The model under review builds one solid part; all positions refer to its coordinate system, in mm. A direction names the side the tool comes from. Give positions to 0.01 mm unless a question says otherwise; leave off trailing zeros. Order: outer loops, then holes, each group sorted by start corner. A loop starts at its lowest first (then second) coordinate and runs counter-clockwise, first axis right, second up. Notation, with made-up numbers: (-33, -3) - (14, -3) arc R31 ccw to (14, 24) - close; hole circle Ø11 at (-38.75, -7). An arc over 180 degrees is marked (long way). Use CSV: the item, a comma, the result in double quotes.
```python
from build123d import *

# Parameters (mm, degrees)
SKETCH1_W           = 56.05
SKETCH1_H           = 61.05
SKETCH1_W_2         = 50.05
SKETCH1_H_2         = 55.05
SKETCH1_W_3         = 44.05
SKETCH1_H_3         = 49.05
BOSS_EXTRUDE1_DEPTH = 3
SKETCH1_3_W         = 56.05
SKETCH1_3_H         = 61.05
SKETCH1_3_W_2       = 50.05
SKETCH1_3_H_2       = 55.05
SKETCH1_3_W_3       = 44.05
SKETCH1_3_H_3       = 49.05
BOSS_EXTRUDE2_DEPTH = 15
SKETCH1_4_W         = 50.05
SKETCH1_4_H         = 55.05
SKETCH1_4_W_2       = 44.05
SKETCH1_4_H_2       = 49.05
BOSS_EXTRUDE3_DEPTH = 18
FILLET1_R           = 2
SKETCH2_R           = 13.25
CUT_EXTRUDE1_DEPTH  = 19
SKETCH2_9_R         = 2.825
SKETCH2_9_R_2       = 1.6
SKETCH2_9_R_3       = 13.25
CUT_EXTRUDE2_DEPTH  = 3
CUT_EXTRUDE3_START  = -3
SKETCH2_10_R        = 1.6
SKETCH2_10_W        = 13
SKETCH2_10_H        = 10.44
SKETCH2_10_H_2      = 1
SKETCH2_10_W_2      = 0.1
SKETCH2_10_H_3      = 11.1
CUT_EXTRUDE3_DEPTH  = 16
SKETCH5_W           = 44.05
SKETCH5_H           = 49.05
CUT_EXTRUDE4_DEPTH  = 1.6
SKETCH2_11_W        = 2.25
SKETCH2_11_H        = 0.408076211
SKETCH2_11_W_2      = 1.5
SKETCH2_11_H_2      = 2.5
CUT_EXTRUDE5_DEPTH  = 1.6


with BuildPart() as part:
    # Sketch1 → Boss-Extrude1 (new body)
    with BuildSketch(Plane(origin=(0, 0, 0), x_dir=(1, 0, 0), z_dir=(0, 1, 0))):
        Rectangle(SKETCH1_W, SKETCH1_H)
        Rectangle(SKETCH1_W_2, SKETCH1_H_2, mode=Mode.SUBTRACT)
        Rectangle(SKETCH1_W_2, SKETCH1_H_2)
        Rectangle(SKETCH1_W_3, SKETCH1_H_3, mode=Mode.SUBTRACT)
        Rectangle(SKETCH1_W_3, SKETCH1_H_3)
    extrude(amount=-BOSS_EXTRUDE1_DEPTH)

    # Sketch1_3 → Boss-Extrude2 (add)
    with BuildSketch(Plane(origin=(0, 0, 0), x_dir=(1, 0, 0), z_dir=(0, 1, 0))):
        Rectangle(SKETCH1_3_W, SKETCH1_3_H)
        Rectangle(SKETCH1_3_W_2, SKETCH1_3_H_2, mode=Mode.SUBTRACT)
        Rectangle(SKETCH1_3_W_2, SKETCH1_3_H_2)
        Rectangle(SKETCH1_3_W_3, SKETCH1_3_H_3, mode=Mode.SUBTRACT)
        Rectangle(SKETCH1_3_W_3, SKETCH1_3_H_3)
    extrude(amount=-BOSS_EXTRUDE2_DEPTH)

    # Sketch1_4 → Boss-Extrude3 (add)
    with BuildSketch(Plane(origin=(0, 0, 0), x_dir=(1, 0, 0), z_dir=(0, 1, 0))):
        Rectangle(SKETCH1_4_W, SKETCH1_4_H)
        Rectangle(SKETCH1_4_W_2, SKETCH1_4_H_2, mode=Mode.SUBTRACT)
    extrude(amount=-BOSS_EXTRUDE3_DEPTH)

    # Fillet1
    fillet1_edges = [part.edges().sort_by_distance(p)[0] for p in [
        (-28.025, 0, 0),
        (0, 0, -30.525),
        (28.025, 0, 0),
        (0, 0, 30.525),
        (-28.025, -7.5, 30.525),
        (-28.025, -7.5, -30.525),
        (28.025, -7.5, -30.525),
        (28.025, -7.5, 30.525),
    ]]
    fillet(fillet1_edges, radius=FILLET1_R)

    # Sketch2 → Cut-Extrude1 (cut, through all)
    with BuildSketch(Plane(origin=(0, 0, 0), x_dir=(1, 0, 0), z_dir=(0, 1, 0))):
        with Locations(Location((-1.25, 0, 0), (0, 0, 270))):  # turned: the seam where the file's is
            Circle(SKETCH2_R)
    extrude(amount=-CUT_EXTRUDE1_DEPTH, mode=Mode.SUBTRACT)

    # Sketch2_9 → Cut-Extrude2 (cut)
    with BuildSketch(Plane(origin=(0, 0, 0), x_dir=(1, 0, 0), z_dir=(0, 1, 0))):
        with Locations(Location((-10.125, 13.665, 0), (0, 0, 270))):  # turned: the seam where the file's is
            Circle(SKETCH2_9_R)
        with Locations((-10.125, 13.665)):
            Circle(SKETCH2_9_R_2, mode=Mode.SUBTRACT)
        with Locations(Location((9.625, 13.665, 0), (0, 0, 270))):  # turned: the seam where the file's is
            Circle(SKETCH2_9_R)
        with Locations((9.625, 13.665)):
            Circle(SKETCH2_9_R_2, mode=Mode.SUBTRACT)
        with Locations(Location((9.625, -12.485, 0), (0, 0, 270))):  # turned: the seam where the file's is
            Circle(SKETCH2_9_R)
        with Locations((9.625, -12.485)):
            Circle(SKETCH2_9_R_2, mode=Mode.SUBTRACT)
        with Locations(Location((-1.25, 0, 0), (0, 0, 270))):  # turned: the seam where the file's is
            Circle(SKETCH2_9_R_3)
        with Locations((-10.125, -12.485)):
            Circle(SKETCH2_9_R)
        with Locations((-10.125, -12.485)):
            Circle(SKETCH2_9_R_2, mode=Mode.SUBTRACT)
        with Locations(Location((-1.25, 0, 0), (0, 0, 270))):  # turned: the seam where the file's is
            Circle(SKETCH2_9_R_3)
        with Locations((-10.125, -12.485)):
            Circle(SKETCH2_9_R)
        with Locations((-10.125, 13.665)):
            Circle(SKETCH2_9_R_2)
        with Locations((9.625, 13.665)):
            Circle(SKETCH2_9_R_2)
        with Locations((9.625, -12.485)):
            Circle(SKETCH2_9_R_2)
        with Locations((-10.125, -12.485)):
            Circle(SKETCH2_9_R_2)
    extrude(amount=-CUT_EXTRUDE2_DEPTH, mode=Mode.SUBTRACT)

    # Sketch2_10 → Cut-Extrude3 (cut, through all)
    with BuildSketch(Plane(origin=(0, 0, 0), x_dir=(1, 0, 0), z_dir=(0, 1, 0)).offset(CUT_EXTRUDE3_START)):
        with Locations(Location((-10.125, 13.665, 0), (0, 0, 270))):  # turned: the seam where the file's is
            Circle(SKETCH2_10_R)
        with Locations(Location((9.625, 13.665, 0), (0, 0, 270))):  # turned: the seam where the file's is
            Circle(SKETCH2_10_R)
        with Locations(Location((9.625, -12.485, 0), (0, 0, 270))):  # turned: the seam where the file's is
            Circle(SKETCH2_10_R)
        with Locations(Location((-10.125, -12.485, 0), (0, 0, 270))):  # turned: the seam where the file's is
            Circle(SKETCH2_10_R)
        with BuildLine():
            Line((-7.125, -17.085), (5.875, -17.085))
            Line((5.875, -17.085), (5.875, -11.171252168))
            ThreePointArc((5.875, -11.171252168), (-0.532432127, -13.230555406), (-7.125, -11.876315717))
            Line((-7.125, -11.876315717), (-7.125, -17.085))
        make_face()
        with Locations((-0.625, -22.305)):
            Rectangle(SKETCH2_10_W, SKETCH2_10_H)
        with Locations((-0.625, -28.025)):
            Rectangle(SKETCH2_10_W, SKETCH2_10_H_2)
        with BuildLine():
            Line((10.781624994, -5.55), (13.25, -5.55))
            Line((13.25, -5.55), (13.25, 5.55))
            Line((13.25, 5.55), (10.781624994, 5.55))
            ThreePointArc((10.781624994, 5.55), (11.691822344, 2.841079797), (12, 0))
            ThreePointArc((12, 0), (11.691822344, -2.841079797), (10.781624994, -5.55))
        make_face()
        with Locations((13.3, 0)):
            Rectangle(SKETCH2_10_W_2, SKETCH2_10_H_3)
    extrude(amount=-CUT_EXTRUDE3_DEPTH, mode=Mode.SUBTRACT)

    # Sketch5 → Cut-Extrude4 (cut)
    with BuildSketch(Plane.XZ.offset(15)):
        Rectangle(SKETCH5_W, SKETCH5_H)
    extrude(amount=-CUT_EXTRUDE4_DEPTH, mode=Mode.SUBTRACT)

    # Sketch2_11 → Cut-Extrude5 (cut)
    with BuildSketch(Plane(origin=(0, 0, 0), x_dir=(1, 0, 0), z_dir=(0, 1, 0))):
        Polygon((-0.375, 27.183076211), (1.125, 27.183076211), (1.125, 27.525), (-1.125, 27.525), (-1.125, 24.183076211), (-0.375, 24.183076211), (-0.375, 25.683076211), (0.375, 25.683076211), (0.375, 26.433076211), (-0.375, 26.433076211), align=None)
        with Locations((0, 27.729038106)):
            Rectangle(SKETCH2_11_W, SKETCH2_11_H)
        Polygon((-1.5, 21.085), (-0.75, 21.085), (0.75, 21.085), (1.5, 21.085), (0, 23.683076211), align=None)
        with Locations((0, 19.835)):
            Rectangle(SKETCH2_11_W_2, SKETCH2_11_H_2)
    extrude(amount=-CUT_EXTRUDE5_DEPTH, mode=Mode.SUBTRACT)


solid = part.part
```
Item 1: Wall thickness on L1, parallel to X at y = -7, z = 12.5 (3 decimals); L2, parallel to X at y = -15.75, z = 16 (3 decimals); L3, parallel to X at y = -12.25, z = 21 (3 decimals): over which ranges is each line inside the solid? List them lowest first.
Results list:
L1,"x = -28.025 to -11.725, -8.525 to -7.125, 5.875 to 8.025, 11.225 to 28.025"
L2,"x = -25.025 to -22.025, 22.025 to 25.025"
L3,"x = -28.025 to -7.125, 5.875 to 28.025"
Item 2: Mouldability with a two-part tool opening along Z and no side actions: class faces 4 (the face through (27.424, -0.57, -0.399)), 5 (the face through (-0.75, -1, -20)), 6 (the face through (0, -8, -30.525)) as pulls with the +Z half, pulls with the -Z half, needs draft (parallel to the pull), parting line crosses it, or undercut.
Results list:
face 4,"needs draft"
face 5,"undercut"
face 6,"pulls with the -Z half"
Item 3: Take a section at A-A, the plane z = 0. Give the boundary of the cut face in (x, y) (3 decimals).
Results list:
outline,"(-28.025, -15) - (-25.025, -15) - (-25.025, -18) - (-22.025, -18) - (-22.025, -13.4) - (-14.5, -13.4) - (-14.5, 0) - (-26.025, 0) arc R2 ccw to (-28.025, -2) - close; (12, -3) - (13.35, -3) - (13.35, -13.4) - (22.025, -13.4) - (22.025, -18) - (25.025, -18) - (25.025, -15) - (28.025, -15) - (28.025, -2) arc R2 ccw to (26.025, 0) - (12, 0) - close"
Item 4: Clearance check with flat-ended pins moving along their axes: pin 1 (10 mm diameter, centred on x = -15, z = -3, fed in from -Y); pin 2 (4 mm diameter, centred on x = 9.625, z = -13.665, fed in from +Y); pin 3 (3 mm diameter, centred on x = -10.125, z = 12.485, fed in from +Y); pin 4 (0.6 mm diameter, centred on x = 1, y = -1, fed in from -Z). State where each tip first meets the part, or that it passes through.
Results list:
pin 1,"stops at y = -13.4"
pin 2,"stops at y = -3"
pin 3,"passes through"
pin 4,"stops at z = -30.4"
Item 5: Take a section at B-B, the plane x = -2.5. Give the boundary of the cut face in (y, z) (3 decimals).
Results list:
outline,"(-18, -27.525) - (-15, -27.525) - (-15, -30.525) - (-2, -30.525) arc R2 ccw to (0, -28.525) - (0, -13.191) - (-13.4, -13.191) - (-13.4, -24.525) - (-18, -24.525) - close; (-15, 28.525) - (-3, 28.525) - (-3, 13.191) - (0, 13.191) - (0, 28.525) arc R2 ccw to (-2, 30.525) - (-15, 30.525) - close"
Item 6: Take a section at D-D, the plane x = -16. Give the boundary of the cut face in (y, z) (3 decimals).
Results list:
outline,"(-18, -27.525) - (-15, -27.525) - (-15, -30.525) - (-2, -30.525) arc R2 ccw to (0, -28.525) - (0, 28.525) arc R2 ccw to (-2, 30.525) - (-15, 30.525) - (-15, 27.525) - (-18, 27.525) - (-18, 24.525) - (-13.4, 24.525) - (-13.4, -24.525) - (-18, -24.525) - close"
Item 7: Tool access review of faces 1 (the face through (-10, -13.4, -11)), 2 (the face through (0.76, -0.79, -22.37)), 3 (the face through (27.424, -8.409, 29.955)): name each direction out of +Z, -Z, +X, -X, +Y, -Y from which nothing blocks a thin tool from reaching the whole face with its end or side.
Results list:
face 1,"-Y"
face 2,"+Y"
face 3,"+Z, +X, +Y, -Y"
Item 8: Take a section at C-C, the plane z = 16.5. Give the boundary of the cut face in (x, y) (3 decimals).
Results list:
outline,"(-28.025, -15) - (-25.025, -15) - (-25.025, -18) - (-22.025, -18) - (-22.025, -13.4) - (-7.125, -13.4) - (-7.125, -3) - (5.875, -3) - (5.875, -13.4) - (22.025, -13.4) - (22.025, -18) - (25.025, -18) - (25.025, -15) - (28.025, -15) - (28.025, -2) arc R2 ccw to (26.025, 0) - (-26.025, 0) arc R2 ccw to (-28.025, -2) - close"
